from build123d import *

# Parameters (mm, degrees)
SKETCH_W        = 150
SKETCH_H        = 79
PAD_DEPTH       = 45
SKETCH001_W     = 144
SKETCH001_H     = 73
POCKET_DEPTH    = 42
SKETCH002_W     = 14.663201
SKETCH002_H     = 6.203663
SKETCH002_W_2   = 16.919073
SKETCH002_H_2   = 8.741524
SKETCH002_W_3   = 14.945191
SKETCH002_H_3   = 5.639692
POCKET001_DEPTH = 3
SKETCH003_R     = 5.949199
SKETCH003_R_2   = 2.588926
SKETCH003_R_3   = 5.354286
SKETCH003_R_4   = 2.696955
SKETCH003_R_5   = 6.584553
SKETCH003_R_6   = 2.878425
PAD001_DEPTH    = 10
POCKET002_DEPTH = 3
SKETCH005_R     = 2.662532
POCKET003_DEPTH = 3


with BuildPart() as part:
    # Sketch → Pad (new body)
    with BuildSketch(Plane.XY):
        Rectangle(SKETCH_W, SKETCH_H)
    extrude(amount=-PAD_DEPTH)

    # Sketch001 → Pocket (cut)
    with BuildSketch(Plane.XY):
        Rectangle(SKETCH001_W, SKETCH001_H)
    extrude(amount=-POCKET_DEPTH, mode=Mode.SUBTRACT)

    # Sketch002 (on DatumPlane) → Pocket001 (cut)
    with BuildSketch(Plane.XZ.offset(39.5)):
        with Locations((-27.918567, -15.816674)):
            Rectangle(SKETCH002_W, SKETCH002_H)
        with Locations((23.966603, -21.879343)):
            Rectangle(SKETCH002_W_2, SKETCH002_H_2)
        with Locations((-2.680947, -31.607812)):
            Rectangle(SKETCH002_W_3, SKETCH002_H_3)
    extrude(amount=-POCKET001_DEPTH, mode=Mode.SUBTRACT)

    # Sketch003 (on DatumPlane) → Pad001 (join)
    with BuildSketch(Plane.XY.offset(-42)):
        with Locations((-33.910699, 18.155216)):
            Circle(SKETCH003_R)
        with Locations((-33.910699, 18.155216)):
            Circle(SKETCH003_R_2, mode=Mode.SUBTRACT)
        with Locations((-35.593381, -9.60911)):
            Circle(SKETCH003_R_3)
        with Locations((-35.593381, -9.60911)):
            Circle(SKETCH003_R_4, mode=Mode.SUBTRACT)
        with Locations((32.979031, 17.313114)):
            Circle(SKETCH003_R_5)
        with Locations((32.979031, 17.313114)):
            Circle(SKETCH003_R_6, mode=Mode.SUBTRACT)
    extrude(amount=PAD001_DEPTH)

    # Sketch004 (on DatumPlane) → Pocket002 (cut)
    with BuildSketch(Plane.XY.offset(-42)):
        with BuildLine():
            ThreePointArc((31.442511, -11.927483), (36.580599, -6.789395), (31.442511, -1.651307))
            Line((31.442511, -1.651307), (10.376326, -1.651307))
            ThreePointArc((10.376326, -1.651307), (5.238238, -6.789395), (10.376326, -11.927483))
            Line((31.442511, -11.927483), (10.376326, -11.927483))
        make_face()
        with BuildLine():
            ThreePointArc((31.95632, -22.717489), (34.525381, -20.148428), (31.95632, -17.579367))
            Line((31.95632, -17.579367), (5.752032, -17.579367))
            ThreePointArc((5.752032, -17.579367), (3.182971, -20.148428), (5.752032, -22.717489))
            Line((31.95632, -22.717489), (5.752032, -22.717489))
        make_face()
    extrude(amount=-POCKET002_DEPTH, mode=Mode.SUBTRACT)

    # Sketch005 (on DatumPlane) → Pocket003 (cut)
    with BuildSketch(Plane.YZ.offset(75)):
        with Locations((-17.169722, -13.141008)):
            Circle(SKETCH005_R)
        with Locations((-9.896163, -13.141008)):
            Circle(SKETCH005_R)
        with Locations((-2.622604, -13.141008)):
            Circle(SKETCH005_R)
        with Locations((4.650955, -13.141008)):
            Circle(SKETCH005_R)
        with Locations((-17.169722, -20.414567)):
            Circle(SKETCH005_R)
        with Locations((-9.896163, -20.414567)):
            Circle(SKETCH005_R)
        with Locations((-2.622604, -20.414567)):
            Circle(SKETCH005_R)
        with Locations((4.650955, -20.414567)):
            Circle(SKETCH005_R)
        with Locations((-17.169722, -27.688126)):
            Circle(SKETCH005_R)
        with Locations((-9.896163, -27.688126)):
            Circle(SKETCH005_R)
        with Locations((-2.622604, -27.688126)):
            Circle(SKETCH005_R)
        with Locations((4.650955, -27.688126)):
            Circle(SKETCH005_R)
    extrude(amount=-POCKET003_DEPTH, mode=Mode.SUBTRACT)


solid = part.part
The listing builds one solid part. Answer for the finished solid, in the listing's coordinates (mm). A direction names the side the tool comes from. Give positions to 0.01 mm unless a question says otherwise; leave off trailing zeros. Write each loop counter-clockwise with the first axis right and the second up, starting at its lowest first coordinate (ties: lowest second). Pieces come first, ordered by that corner, then holes. Notation, with made-up numbers: (-1, 87) - (53, 87) arc R19 cw to (53, 104) - close; hole circle Ø9 at (-37.5, 77). An arc over 180 degrees is marked (long way). One line per question, with ' | ' between items. Start each with the question number.
1. Given P1, Ø3, axis at y = -2.62, z = -20.41, coming from the +X side; P2, Ø6.5, axis at x = 33, y = 18.5, coming from the +Z side; P3, Ø3, axis at x = 57.5, y = 8, coming from the +Z side, each flat-ended and moving along its own axis, determine where each tip first touches the part or whether it passes through.
2. Section B-B, the plane x = 46.5 is taken. Determine the outline of the cut face in (y, z), then the cut area to 3 significant figures.
3. Section A-A, the plane z = -3 is taken. Determine the outline of the cut face in (x, y).
4. Section C-C, the plane x = -25 is taken. Determine the outline of the cut face in (y, z), then the cut area to 3 significant figures.
5. Determine the mould class of faces 1 (the face through (-1, -39.5, -22)), 2 (the face through (-34.685, 24.054, -37.07)), 3 (the face through (24, -38, -17.509)) for opening direction Y: +Y half, -Y half, draft (parallel to the pull), parting line (faces both ways), or undercut.
6. For faces 4 (the face through (-34, 18, -42)), 5 (the face through (73.52, 4.3, -25.05)), 6 (the face through (19, -22.717, -43)), 7 (the face through (4.792, -38, -32)), determine the directions among +Z, -Z, +X, -X, +Y, -Y from which every point of the face is accessible in a straight line to the end or side of a thin tool.
7. Straight lines are drawn through the part: line 1 (X direction, y = -36, z = -14.5); line 2 (Y direction, x = -43, z = -10.5); line 3 (X direction, y = 7, z = -14). For each, find the intervals that lie inside material, in ascending order.
8. Section D-D, the plane z = -36.5 is taken. Determine the outline of the cut face in (x, y), then the cut area to 3 significant figures.
Result:
1) P1: stops at x = -72 | P2: stops at z = -32 | P3: stops at z = -42
2) outline: (-39.5, -45) - (39.5, -45) - (39.5, 0) - (36.5, 0) - (36.5, -42) - (-36.5, -42) - (-36.5, 0) - (-39.5, 0) - close | area: 489 mm2
3) outline: (-75, -39.5) - (75, -39.5) - (75, 39.5) - (-75, 39.5) - close; hole (-72, -36.5) - (72, -36.5) - (72, 36.5) - (-72, 36.5) - close
4) outline: (-39.5, -45) - (39.5, -45) - (39.5, 0) - (36.5, 0) - (36.5, -42) - (-36.5, -42) - (-36.5, -18.92) - (-39.5, -18.92) - close; (-39.5, -12.71) - (-36.5, -12.71) - (-36.5, 0) - (-39.5, 0) - close | area: 470 mm2
5) face 1: -Y half | face 2: undercut | face 3: draft
6) face 4: +Z | face 5: +X | face 6: +Z, -Z | face 7: -Y
7) line 1: x = -75 to -72, 72 to 75 | line 2: y = -39.5 to -36.5, 36.5 to 39.5 | line 3: x = -75 to -72
8) outline: (-75, -39.5) - (75, -39.5) - (75, 39.5) - (-75, 39.5) - close; circle Ø10.71 at (-35.59, -9.61); circle Ø11.9 at (-33.91, 18.16); circle Ø13.17 at (32.98, 17.31); hole (-72, -36.5) - (72, -36.5) - (72, 36.5) - (-72, 36.5) - close; hole circle Ø5.39 at (-35.59, -9.61); hole circle Ø5.18 at (-33.91, 18.16); hole circle Ø5.76 at (32.98, 17.31) | area: 1,610 mm2
